from build123d import *

# Parameters (mm, degrees)
SKETCH_1_R      = 38.5
EXTRUDE_1_DEPTH = 51
SKETCH_2_R      = 6
EXTRUDE_2_DEPTH = 15


with BuildPart() as part:
    # 草图1 → 凸台-拉伸1 (new, symmetric)
    with BuildSketch(Plane(origin=(0, 0, 0), x_dir=(1, 0, 0), z_dir=(0, 1, 0))):
        with Locations(Location((0, 0, 0), (0, 0, 270))):
            Circle(SKETCH_1_R)
    extrude(amount=EXTRUDE_1_DEPTH, both=True)

    # 草图2 → 凸台-拉伸2 (add)
    with BuildSketch(Plane(origin=(0, 51, 0), x_dir=(1, 0, 0), z_dir=(0, 1, 0))):
        with Locations(Location((16, 0, 0), (0, 0, 270))):
            Circle(SKETCH_2_R)
        with Locations(Location((-16, 0, 0), (0, 0, 90))):
            Circle(SKETCH_2_R)
    extrude(amount=EXTRUDE_2_DEPTH)


solid = part.part
Source: CAD feature listing. Evaluate the final solid. Frame: model axes, mm. Coordinates: 2 decimals unless noted, no trailing zeros. Loops run counter-clockwise (first coordinate to the right, second up) from the corner with the lowest first, then second, coordinate; pieces in that order, holes last. Notation, with made-up numbers: (-7, -3.75) - (16, -3.75) arc R21 ccw to (16, 4.25) - close; hole circle Ø10 at (-21, 31.5). An arc over 180 degrees is marked (long way). One line per item, written item: value. Start each with the question number.
1. Section A-A (z = 0). Return the cut outline in (x, y).
2. Ray query, L1, parallel to Y at x = -27, z = 4; L2, parallel to Z at x = 0.5, y = -3; L3, parallel to Z at x = 30, y = -2.5. Return the intervals inside material, ascending.
3. Section C-C (y = 4). Return the cut outline in (x, z), and give its area (3 significant figures).
4. Contact query for flat-ended pins moving along their axis: P1, Ø1.5, axis at x = -6.5, y = 34.5, coming from the +Z side; P2, Ø5, axis at x = 20, y = -36.5, coming from the -Z side; P3, Ø1, axis at y = 10, z = 10, coming from the +X side. Output: stop coordinate, or through.
5. Mould query, pull axis X, two halves, no side actions, for faces 1 (the cylindrical face through (-37.584, 0.714, -8.346)), 2 (the cylindrical face through (17.802, 58.395, 5.723)), 3 (the cylindrical face through (-17.802, 58.395, -5.723)), 4 (the flat face through (-16, 66, 0)). Classes: pulls with the +X half, pulls with the -X half, needs draft (parallel to the pull), parting line crosses it, or undercut.
6. Section B-B (x = -16). Return the cut outline in (y, z), and give its area (3 significant figures).
7. Section D-D (x = 18). Return the cut outline in (y, z).
Verdict:
1. outline: (-38.5, -51) - (38.5, -51) - (38.5, 51) - (22, 51) - (22, 66) - (10, 66) - (10, 51) - (-10, 51) - (-10, 66) - (-22, 66) - (-22, 51) - (-38.5, 51) - close
2. L1: y = -51 to 51
2. L2: z = -38.5 to 38.5
2. L3: z = -24.13 to 24.13
3. outline: circle Ø77 at (0, 0)
3. area: 4,660 mm2
4. P1: stops at z = 38.07
4. P2: stops at z = -34.29
4. P3: stops at x = 37.31
5. face 1: parting line crosses it
5. face 2: undercut
5. face 3: undercut
5. face 4: needs draft
6. outline: (-51, -35.02) - (51, -35.02) - (51, -6) - (66, -6) - (66, 6) - (51, 6) - (51, 35.02) - (-51, 35.02) - close
6. area: 7,320 mm2
7. outline: (-51, -34.03) - (51, -34.03) - (51, -5.66) - (66, -5.66) - (66, 5.66) - (51, 5.66) - (51, 34.03) - (-51, 34.03) - close
